Geometry check sheet. Reference: the model listing, model coordinates, mm. A direction names the side the tool comes from. Coordinates: 2 decimals unless noted, no trailing zeros. Loops run counter-clockwise (first coordinate to the right, second up) from the corner with the lowest first, then second, coordinate; pieces in that order, holes last. Notation, with made-up numbers: (87, 4.5) - (128, 4.5) arc R9 cw to (128, 8.5) - close; hole circle Ø6 at (25, 43.5). An arc over 180 degrees is marked (long way). One line per item, written item: value.
from build123d import *

# Parameters (mm, degrees)
BASE_FLANGE1_DEPTH             = 104
EDGE_FLANGE1_STRIP_W           = 6
EDGE_FLANGE1_STRIP_H           = 1
EDGE_FLANGE1_STRIP_CUT_DEPTH   = 821.4
EDGE_FLANGE1_RELIEF_W          = 6.5
EDGE_FLANGE1_RELIEF_H          = 0.5
EDGE_FLANGE1_RELIEF_CUT_DEPTH  = 1
EDGE_FLANGE1_DEPTH             = 821.4
EDGE_FLANGE2_STRIP_W           = 6
EDGE_FLANGE2_STRIP_H           = 1
EDGE_FLANGE2_STRIP_CUT_DEPTH   = 821.4
EDGE_FLANGE2_DEPTH             = 821.4
EDGE_FLANGE3_STRIP_W           = 6
EDGE_FLANGE3_STRIP_H           = 1
EDGE_FLANGE3_STRIP_CUT_DEPTH   = 80
EDGE_FLANGE3_RELIEF_W          = 6.5
EDGE_FLANGE3_RELIEF_H          = 0.5
EDGE_FLANGE3_RELIEF_CUT_DEPTH  = 1
EDGE_FLANGE3_DEPTH             = 80
EDGE_FLANGE4_STRIP_W           = 6
EDGE_FLANGE4_STRIP_H           = 1
EDGE_FLANGE4_STRIP_CUT_DEPTH   = 80
EDGE_FLANGE4_DEPTH             = 80
EDGE_FLANGE5_STRIP_W           = 6
EDGE_FLANGE5_STRIP_H           = 1
EDGE_FLANGE5_STRIP_CUT_DEPTH   = 421.4
EDGE_FLANGE5_RELIEF_W          = 6.5
EDGE_FLANGE5_RELIEF_H          = 0.5
EDGE_FLANGE5_RELIEF_CUT_DEPTH  = 1
EDGE_FLANGE5_DEPTH             = 421.4
SKETCH22_R                     = 2.5
CUT_EXTRUDE1_DEPTH             = 1
SKETCH23_R                     = 2.5
CUT_EXTRUDE2_DEPTH             = 3
CUT_EXTRUDE2_DIRECTION_2_REACH = 857.652
EDGE_FLANGE6_STRIP_W           = 6
EDGE_FLANGE6_STRIP_H           = 1
EDGE_FLANGE6_STRIP_CUT_DEPTH   = 421.4
EDGE_FLANGE6_DEPTH             = 421.4
EDGE_FLANGE6_FLAT_DEPTH        = 1


# Sheet-metal steps are written as plain solids
with BuildPart() as part:
    # Sketch1 → Base-Flange1 (new body)
    with BuildSketch(Plane.XY):
        with BuildLine():
            Line((-430.7, -100), (-430.7, -15))
            ThreePointArc((-430.7, -15), (-426.306601718, -4.393398282), (-415.7, 0))
            Line((-415.7, 0), (415.7, 0))
            ThreePointArc((415.7, 0), (426.306601718, -4.393398282), (430.7, -15))
            Line((430.7, -15), (430.7, -100))
            Line((430.7, -100), (431.7, -100))
            Line((431.7, -100), (431.7, -15))
            ThreePointArc((431.7, -15), (427.013708499, -3.686291501), (415.7, 1))
            Line((415.7, 1), (-415.7, 1))
            ThreePointArc((-415.7, 1), (-427.013708499, -3.686291501), (-431.7, -15))
            Line((-431.7, -15), (-431.7, -100))
            Line((-431.7, -100), (-430.7, -100))
        make_face()
    extrude(amount=BASE_FLANGE1_DEPTH)

    # Edge-Flange1 strip (across the edge) → Edge-Flange1 strip cut (cut)
    with BuildSketch(Plane(origin=(-410.7, 0, 0), x_dir=(0, 0, 1), z_dir=(1, 0, 0))):
        with Locations((-2, -0.5)):
            Rectangle(EDGE_FLANGE1_STRIP_W, EDGE_FLANGE1_STRIP_H)
    extrude(amount=EDGE_FLANGE1_STRIP_CUT_DEPTH, mode=Mode.SUBTRACT)

    # Edge-Flange1 relief (on the sheet) → Edge-Flange1 relief cut (cut)
    with BuildSketch(Plane(origin=(-410.7, 0, 1), x_dir=(0, 0, 1), z_dir=(0, -1, 0))):
        with Locations((-2.75, 0.25)):
            Rectangle(EDGE_FLANGE1_RELIEF_W, EDGE_FLANGE1_RELIEF_H)
        with Locations((-2.75, -821.65)):
            Rectangle(EDGE_FLANGE1_RELIEF_W, EDGE_FLANGE1_RELIEF_H)
    extrude(amount=-EDGE_FLANGE1_RELIEF_CUT_DEPTH, mode=Mode.SUBTRACT)

    # Edge-Flange1 section (across the edge) → Edge-Flange1 (add)
    with BuildSketch(Plane(origin=(-410.7, 0, 0), x_dir=(0, 0, 1), z_dir=(1, 0, 0))):
        with BuildLine():
            Line((-1, 1), (-1, 19))
            Line((-1, 19), (0, 19))
            Line((0, 19), (0, 1))
            ThreePointArc((0, 1), (0.292893219, 0.292893219), (1, 0))
            Line((1, 0), (1, -1))
            ThreePointArc((1, -1), (-0.414213562, -0.414213562), (-1, 1))
        make_face()
    extrude(amount=EDGE_FLANGE1_DEPTH)

    # Edge-Flange2 strip (across the edge) → Edge-Flange2 strip cut (cut)
    with BuildSketch(Plane(origin=(-410.7, -19, 0), x_dir=(0, 1, 0), z_dir=(1, 0, 0))):
        with Locations((-1, -0.5)):
            Rectangle(EDGE_FLANGE2_STRIP_W, EDGE_FLANGE2_STRIP_H)
    extrude(amount=EDGE_FLANGE2_STRIP_CUT_DEPTH, mode=Mode.SUBTRACT)

    # Edge-Flange2 section (across the edge) → Edge-Flange2 (add)
    with BuildSketch(Plane(origin=(-410.7, -19, 0), x_dir=(0, 1, 0), z_dir=(1, 0, 0))):
        with BuildLine():
            Line((0, 1), (0, 12))
            Line((0, 12), (1, 12))
            Line((1, 12), (1, 1))
            ThreePointArc((1, 1), (1.292893219, 0.292893219), (2, 0))
            Line((2, 0), (2, -1))
            ThreePointArc((2, -1), (0.585786438, -0.414213562), (0, 1))
        make_face()
    extrude(amount=EDGE_FLANGE2_DEPTH)

    # Edge-Flange3 strip (across the edge) → Edge-Flange3 strip cut (cut)
    with BuildSketch(Plane(origin=(-430.7, -100, 0), x_dir=(0, 0, 1), z_dir=(0, 1, 0))):
        with Locations((-2, -0.5)):
            Rectangle(EDGE_FLANGE3_STRIP_W, EDGE_FLANGE3_STRIP_H)
    edge_flange3_strip_cut = extrude(amount=EDGE_FLANGE3_STRIP_CUT_DEPTH, mode=Mode.SUBTRACT)

    # Edge-Flange3 relief (on the sheet) → Edge-Flange3 relief cut (cut)
    with BuildSketch(Plane(origin=(-430.7, -100, 1), x_dir=(0, 0, 1), z_dir=(1, 0, 0))):
        with Locations((-2.75, -80.25)):
            Rectangle(EDGE_FLANGE3_RELIEF_W, EDGE_FLANGE3_RELIEF_H)
    edge_flange3_relief_cut = extrude(amount=-EDGE_FLANGE3_RELIEF_CUT_DEPTH, mode=Mode.SUBTRACT)

    # Edge-Flange3 section (across the edge) → Edge-Flange3 (add)
    with BuildSketch(Plane(origin=(-430.7, -100, 0), x_dir=(0, 0, 1), z_dir=(0, 1, 0))):
        with BuildLine():
            Line((-1, 1), (-1, 19))
            Line((-1, 19), (0, 19))
            Line((0, 19), (0, 1))
            ThreePointArc((0, 1), (0.292893219, 0.292893219), (1, 0))
            Line((1, 0), (1, -1))
            ThreePointArc((1, -1), (-0.414213562, -0.414213562), (-1, 1))
        make_face()
    edge_flange3 = extrude(amount=EDGE_FLANGE3_DEPTH)

    # Edge-Flange4 strip (across the edge) → Edge-Flange4 strip cut (cut)
    with BuildSketch(Plane(origin=(-411.7, -100, 0), x_dir=(-1, 0, 0), z_dir=(0, 1, 0))):
        with Locations((-1, -0.5)):
            Rectangle(EDGE_FLANGE4_STRIP_W, EDGE_FLANGE4_STRIP_H)
    edge_flange4_strip_cut = extrude(amount=EDGE_FLANGE4_STRIP_CUT_DEPTH, mode=Mode.SUBTRACT)

    # Edge-Flange4 section (across the edge) → Edge-Flange4 (add)
    with BuildSketch(Plane(origin=(-411.7, -100, 0), x_dir=(-1, 0, 0), z_dir=(0, 1, 0))):
        with BuildLine():
            Line((0, 1), (0, 12))
            Line((0, 12), (1, 12))
            Line((1, 12), (1, 1))
            ThreePointArc((1, 1), (1.292893219, 0.292893219), (2, 0))
            Line((2, 0), (2, -1))
            ThreePointArc((2, -1), (0.585786438, -0.414213562), (0, 1))
        make_face()
    edge_flange4 = extrude(amount=EDGE_FLANGE4_DEPTH)

    # Mirror1: Edge-Flange3 strip cut, Edge-Flange3 relief cut, Edge-Flange3, Edge-Flange4 strip cut, Edge-Flange4 across plane
    add(edge_flange3_strip_cut.mirror(Plane(origin=(0, 0, 0), x_dir=(0, 0, 1), z_dir=(1, 0, 0))), mode=Mode.SUBTRACT)
    add(edge_flange3_relief_cut.mirror(Plane(origin=(0, 0, 0), x_dir=(0, 0, 1), z_dir=(1, 0, 0))), mode=Mode.SUBTRACT)
    add(edge_flange3.mirror(Plane(origin=(0, 0, 0), x_dir=(0, 0, 1), z_dir=(1, 0, 0))))
    add(edge_flange4_strip_cut.mirror(Plane(origin=(0, 0, 0), x_dir=(0, 0, 1), z_dir=(1, 0, 0))), mode=Mode.SUBTRACT)
    add(edge_flange4.mirror(Plane(origin=(0, 0, 0), x_dir=(0, 0, 1), z_dir=(1, 0, 0))))

    # Edge-Flange5 strip (across the edge) → Edge-Flange5 strip cut (cut)
    with BuildSketch(Plane(origin=(210.7, 0, 104), x_dir=(0, 0, -1), z_dir=(-1, 0, 0))):
        with Locations((-1, -0.5)):
            Rectangle(EDGE_FLANGE5_STRIP_W, EDGE_FLANGE5_STRIP_H)
    extrude(amount=EDGE_FLANGE5_STRIP_CUT_DEPTH, mode=Mode.SUBTRACT)

    # Edge-Flange5 relief (on the sheet) → Edge-Flange5 relief cut (cut)
    with BuildSketch(Plane(origin=(210.7, 0, 102), x_dir=(0, 0, -1), z_dir=(0, -1, 0))):
        with Locations((-2.75, 0.25)):
            Rectangle(EDGE_FLANGE5_RELIEF_W, EDGE_FLANGE5_RELIEF_H)
        with Locations((-2.75, -421.65)):
            Rectangle(EDGE_FLANGE5_RELIEF_W, EDGE_FLANGE5_RELIEF_H)
    extrude(amount=-EDGE_FLANGE5_RELIEF_CUT_DEPTH, mode=Mode.SUBTRACT)

    # Edge-Flange5 section (across the edge) → Edge-Flange5 (add)
    with BuildSketch(Plane(origin=(210.7, 0, 104), x_dir=(0, 0, -1), z_dir=(-1, 0, 0))):
        with BuildLine():
            Line((0, 1), (0, 35.5))
            Line((0, 35.5), (1, 35.5))
            Line((1, 35.5), (1, 1))
            ThreePointArc((1, 1), (1.292893219, 0.292893219), (2, 0))
            Line((2, 0), (2, -1))
            ThreePointArc((2, -1), (0.585786438, -0.414213562), (0, 1))
        make_face()
    extrude(amount=EDGE_FLANGE5_DEPTH)

    # Sketch22 → Cut-Extrude1 (cut)
    with BuildSketch(Plane.XZ.offset(19)):
        with Locations(Location((-349.7, 6, 0), (0, 0, 270))):
            Circle(SKETCH22_R)
        with Locations(Location((-169.7, 6, 0), (0, 0, 270))):
            Circle(SKETCH22_R)
        with Locations(Location((10.3, 6, 0), (0, 0, 270))):
            Circle(SKETCH22_R)
        with Locations(Location((190.3, 6, 0), (0, 0, 270))):
            Circle(SKETCH22_R)
        with Locations(Location((370.3, 6, 0), (0, 0, 270))):
            Circle(SKETCH22_R)
        with Locations((550.3, 6)):
            Circle(SKETCH22_R)
        with Locations((730.3, 6)):
            Circle(SKETCH22_R)
    extrude(amount=-CUT_EXTRUDE1_DEPTH, mode=Mode.SUBTRACT)

    # Sketch23 → Cut-Extrude2 (cut)
    with BuildSketch(Plane.ZY.offset(-411.7)):
        with Locations(Location((6, -68, 0), (0, 0, 180))):
            Circle(SKETCH23_R)
    extrude(amount=-CUT_EXTRUDE2_DEPTH, mode=Mode.SUBTRACT)

    # Cut-Extrude2 direction 2: up to this face of the body (flat: up to its plane)
    cut_extrude2_direction_2_end = Plane(part.part.faces().sort_by_distance((-412.7, -60, 6.5))[0])
    # Sketch23 → Cut-Extrude2 direction 2 (cut, up to the picked face)
    with BuildSketch(Plane.ZY.offset(-411.7), mode=Mode.PRIVATE) as cut_extrude2_direction_2_sk1:
        with Locations(Location((6, -68, 0), (0, 0, 180))):
            Circle(SKETCH23_R)
    cut_extrude2_direction_2_tool1 = split(extrude(cut_extrude2_direction_2_sk1.sketch, amount=CUT_EXTRUDE2_DIRECTION_2_REACH, mode=Mode.PRIVATE), bisect_by=cut_extrude2_direction_2_end, keep=Keep.BOTH, mode=Mode.PRIVATE)
    add(cut_extrude2_direction_2_tool1.solids().sort_by(Axis((411.7, -68, 6), (-1, 0, 0)))[0], mode=Mode.SUBTRACT)

    # Edge-Flange6 strip (across the edge) → Edge-Flange6 strip cut (cut)
    with BuildSketch(Plane(origin=(210.7, -35.5, 103), x_dir=(0, 1, 0), z_dir=(-1, 0, 0))):
        with Locations((-1, -0.5)):
            Rectangle(EDGE_FLANGE6_STRIP_W, EDGE_FLANGE6_STRIP_H)
    extrude(amount=EDGE_FLANGE6_STRIP_CUT_DEPTH, mode=Mode.SUBTRACT)

    # Edge-Flange6 bend section (across the edge) → Edge-Flange6 (add)
    with BuildSketch(Plane(origin=(210.7, -35.5, 103), x_dir=(0, 1, 0), z_dir=(-1, 0, 0))):
        with BuildLine():
            Line((0, 1), (1, 1))
            ThreePointArc((1, 1), (1.292893219, 0.292893219), (2, 0))
            Line((2, 0), (2, -1))
            ThreePointArc((2, -1), (0.585786438, -0.414213562), (0, 1))
        make_face()
    extrude(amount=EDGE_FLANGE6_DEPTH)

    # Edge-Flange6 profile (on flange) → Edge-Flange6 flat (add)
    with BuildSketch(Plane(origin=(0, -35.5, 103), x_dir=(1, 0, 0), z_dir=(0, 1, 0))):
        with BuildLine():
            Line((-210.7, 1), (210.7, 1))
            Line((210.7, 1), (210.7, 11))
            ThreePointArc((210.7, 11), (209.821320344, 13.121320344), (207.7, 14))
            Line((207.7, 14), (-207.7, 14))
            ThreePointArc((-207.7, 14), (-209.821320344, 13.121320344), (-210.7, 11))
            Line((-210.7, 11), (-210.7, 1))
        make_face()
    extrude(amount=EDGE_FLANGE6_FLAT_DEPTH)


solid = part.part
(1) Access from +Z, -Z, +X, -X, +Y, -Y to the whole of each face (thin tool, end or side, straight path). Record for faces 1 (the face through (-426.1, -3.9, 0)), 2 (the face through (-6, -9, 0)), 3 (the face through (427, -4, 0)).
Reply:
face 1: -Z, -X, +Y
face 2: none
face 3: -Z, +X, +Y
(2) Cross-section at B-B on z = 31.5. Record the cut outline in (x, y), and give its area (3 significant figures).
Reply:
outline: (-431.7, -100) - (-430.7, -100) - (-430.7, -15) arc R15 cw to (-415.7, 0) - (415.7, 0) arc R15 cw to (430.7, -15) - (430.7, -100) - (431.7, -100) - (431.7, -15) arc R16 ccw to (415.7, 1) - (-415.7, 1) arc R16 ccw to (-431.7, -15) - close
area: 1,050 mm2
(3) Cross-section at D-D on x = 120. Record the cut outline in (y, z).
Reply:
outline: (-35.5, 89) - (-34.5, 89) - (-34.5, 102) arc R1 cw to (-33.5, 103) - (-1, 103) arc R1 cw to (0, 102) - (0, 1) arc R1 cw to (-1, 0) - (-17, 0) arc R1 cw to (-18, 1) - (-18, 12) - (-19, 12) - (-19, 1) arc R2 ccw to (-17, -1) - (-1, -1) arc R2 ccw to (1, 1) - (1, 102) arc R2 ccw to (-1, 104) - (-33.5, 104) arc R2 ccw to (-35.5, 102) - close
(4) Go/stop test with flat-tipped pins: pin 1 Ø1.1 at (x, y) = (-412.5, -41.5) entering from +Z; pin 2 Ø3 at (x, y) = (175.5, -28.5) entering from -Z; pin 3 Ø1 at (x, z) = (-36.5, 46) entering from -Y. Record where each tip stops, or that it passes through.
Reply:
pin 1: z = 12
pin 2: z = 103
pin 3: y = 0
(5) Cross-section at A-A on y = -58. Record the cut outline in (x, z), and give its area (3 significant figures).
Reply:
outline: (-431.7, 1) arc R2 ccw to (-429.7, -1) - (-413.7, -1) arc R2 ccw to (-411.7, 1) - (-411.7, 12) - (-412.7, 12) - (-412.7, 1) arc R1 cw to (-413.7, 0) - (-429.7, 0) arc R1 cw to (-430.7, 1) - (-430.7, 104) - (-431.7, 104) - close; (411.7, 1) arc R2 ccw to (413.7, -1) - (429.7, -1) arc R2 ccw to (431.7, 1) - (431.7, 104) - (430.7, 104) - (430.7, 1) arc R1 cw to (429.7, 0) - (413.7, 0) arc R1 cw to (412.7, 1) - (412.7, 12) - (411.7, 12) - close
area: 269 mm2
(6) Material ranges on probe 1 along X at (y, z) = (-84, 10); probe 2 along Y at (x, z) = (-412, 6); probe 3 along X at (y, z) = (-56.5, 25), recorded low to high. Write a range as from..to.
Reply:
probe 1: -431.7..-430.7, -412.7..-411.7, 411.7..412.7, 430.7..431.7
probe 2: -100..-70.5, -65.5..-20, 0..1
probe 3: -431.7..-430.7, 430.7..431.7
(7) Release check for a two-part mould opening along Z. For faces 4 (the face through (3, -17, 103)), 5 (the face through (-431, -100, 48)), 6 (the face through (-6, -9, -1)) record: pulls with the +Z half, pulls with the -Z half, needs draft (parallel to the pull), parting line crosses it, or undercut.
Reply:
face 4: undercut
face 5: needs draft
face 6: pulls with the -Z half
(8) Cross-section at C-C on x = -249. Record the cut outline in (y, z), and give its area (3 significant figures).
Reply:
outline: (-19, 1) arc R2 ccw to (-17, -1) - (-1, -1) arc R2 ccw to (1, 1) - (1, 104) - (0, 104) - (0, 1) arc R1 cw to (-1, 0) - (-17, 0) arc R1 cw to (-18, 1) - (-18, 12) - (-19, 12) - close
area: 135 mm2
